Could you check a few things on this model? Use its own coordinates, in mm. A direction names the side the tool comes from. Give positions to 0.01 mm unless a question says otherwise; leave off trailing zeros. Write each loop counter-clockwise with the first axis right and the second up, starting at its lowest first coordinate (ties: lowest second). Pieces come first, ordered by that corner, then holes. Notation, with made-up numbers: (83, 68.5) -> (132, 68.5) arc R19 ccw to (132, 89.5) -> close; hole circle Ø8 at (-26.5, 57). An arc over 180 degrees is marked (long way). One line per question, with ' | ' between items.
Autodesk Inventor part; units mm, degrees
ref_plane "YZ Plane" through (0, 0, 0) normal (1, 0, 0) x (0, 1, 0)
ref_plane "XZ Plane" through (0, 0, 0) normal (0, 1, 0) x (-1, 0, 0)
ref_plane "XY Plane" through (0, 0, 0) normal (0, 0, 1) x (1, 0, 0)
sketch "Sketch5" plane through (0, 0, 0) normal (0, 0, 1) x (1, 0, 0)
  line L0 (59.877, 38.0614) -> (231.327, 38.0614)
  line L1 (231.327, 38.0614) -> (231.327, -7.9761)
  line L2 (231.327, -7.9761) -> (59.877, -7.9761)
  line L3 (59.877, -7.9761) -> (59.877, 38.0614)
  dimension "d28" = 46.0375
  dimension "d29" = 171.45
extrude "Extrusion4" add sketch "Sketch5" along normal blind 139.7
sketch "Sketch6" plane through (0, 0, 139.7) normal (0, 0, 1) x (1, 0, 0)
  line L0 (231.327, 38.0614) -> (231.327, -7.9761)
  line L1 (231.327, -7.9761) -> (59.877, -7.9761)
  line L2 (231.327, -7.9761) -> (-73.473, 30.1239)
  line L3 (-73.473, 30.1239) -> (-73.473, -7.9761)
  line L4 (59.877, -7.9761) -> (-73.473, -7.9761)
  dimension "d32" = 304.8
  dimension "d33" = 38.1
extrude "Extrusion5" cut sketch "Sketch6" against normal through all
sketch "Sketch7" plane through (59.877, 38.0614, 0) normal (0, 1, 0) x (1, 0, 0)
  line L0 (0, -139.7) -> (171.45, -139.7)
  line L1 (0, 0) -> (0, -139.7)
  arc A0 (73.025, -47.625) -> (73.025, -92.075) centre (73.025, -69.85) ccw
  arc A1 (117.475, -92.075) -> (117.475, -47.625) centre (117.475, -69.85) ccw
  line L2 (73.025, -92.075) -> (117.475, -92.075)
  line L3 (73.025, -47.625) -> (117.475, -47.625)
  dimension "d36" = 69.85
  dimension "d37" = 22.225
  dimension "d38" = 73.025
  dimension "d39" = 44.45
extrude "Extrusion6" cut sketch "Sketch7" against normal through all
sketch "Sketch8" plane through (59.877, 38.0614, 0) normal (0, 1, 0) x (1, 0, 0)
  line L0 (0, -139.7) -> (171.45, -139.7)
  line L1 (0, 0) -> (171.45, 0)
  line L2 (0, 0) -> (0, -139.7)
  line L3 (38.1, -139.7) -> (0, -117.703)
  line L4 (0, -21.997) -> (38.1, 0)
  dimension "d42" = 30
  dimension "d43" = 38.1
  dimension "d56" = 30
extrude "Extrusion7" cut sketch "Sketch8" against normal through all
sketch "Sketch9" plane through (231.327, 38.0614, 139.7) normal (1, 0, 0) x (0, 0, -1)
  line L0 (0, 0) -> (0, -46.0375)
  line L1 (139.7, 0) -> (0, 0)
  point P0 (69.85, -25.4)
  dimension "d46" = 69.85
  dimension "d47" = 25.4
hole "Hole2" at (231.327, 12.6614, 69.85) direction (-1, 0, 0) diameter 19.177 end up to surface
fillet "Fillet2" radius 3.175 6 edges at (97.977, 23.377, 139.7) (59.877, 25.7583, 117.703) (59.877, 25.7583, 21.997) (97.977, 23.377, 0) (231.327, 15.0427, 0) (231.327, 15.0427, 139.7)
properties part number "Wedge"
Q1. If I drill on line 1 along Z through (x, y) = (146, 3) (3 decimals); line 2 along Y through (x, z) = (212, 69); line 3 along Y through (x, z) = (215, 69), over which ranges is the centre line in solid material (lowest first)?
Answer below:
line 1: z = 0 to 47.625, 92.075 to 139.7 | line 2: y = -5.56 to 3.11, 22.21 to 38.06 | line 3: y = -5.94 to 3.11, 22.21 to 38.06
Q2. Imagine slicing it at A-A on x = 183.5. Please give me the cut outline in (y, z), and give its area (3 significant figures).
Answer below:
outline: (-2, 0) -> (38.06, 0) -> (38.06, 48.49) -> (-2, 48.49) -> close; (-2, 91.21) -> (38.06, 91.21) -> (38.06, 139.7) -> (-2, 139.7) -> close | area: 3,890 mm^2
Q3. Imagine slicing it at C-C on z = 67. Please give me the cut outline in (x, y).
Answer below:
outline: (59.88, 13.46) -> (110.86, 7.08) -> (110.86, 38.06) -> (59.88, 38.06) -> close; (199.39, -3.98) -> (231.33, -7.98) -> (231.33, 3.51) -> (199.39, 3.51) -> close; (199.39, 21.82) -> (231.33, 21.82) -> (231.33, 38.06) -> (199.39, 38.06) -> close
Q4. On a 3-axis mill with a long thin cutter (end or side, diameter ignored), from which of +Z, -Z, +X, -X, +Y, -Y can I reach the whole of each face in a straight line? I mean faces 1 (the flat face through (155, 19, 47.625)), 2 (the flat face through (79.1, 23.6, 10.9)), 3 (the cylindrical face through (214.127, 3.154, 71.098)). Say none if no direction works.
Answer below:
face 1: +Y, -Y | face 2: -Z, -X, +Y, -Y | face 3: +X
Q5. If we mould it in two halves opening along X, with no side actions, what happens to faces 4 (the flat face through (231.327, 26, 69)), 5 (the flat face through (144, 38.061, 38)), 6 (the flat face through (155, 19, 92.075)), 7 (the flat face through (79.6, 23.63, 129.09))? For each: +X half, -X half, draft (parallel to the pull), parting line (faces both ways), or undercut.
Answer below:
face 4: +X half | face 5: draft | face 6: undercut | face 7: -X half
Q6. Will these pins go through, and if not, where does the flat tip stop? pin 1 (15.5 mm diameter, centred on y = 12.66, z = 69.85, fed in from -X); pin 2 (6 mm diameter, centred on x = 83, z = 124, fed in from -Y); pin 3 (2 mm diameter, centred on x = 163, z = 46, fed in from -Y).
Answer below:
pin 1: stops at x = 59.88 | pin 2: stops at y = 10.19 | pin 3: stops at y = 0.44
Q7. Imagine slicing it at D-D on z = 109. Please give me the cut outline in (x, y).
Answer below:
outline: (59.88, 13.46) -> (231.33, -7.98) -> (231.33, 38.06) -> (59.88, 38.06) -> close
